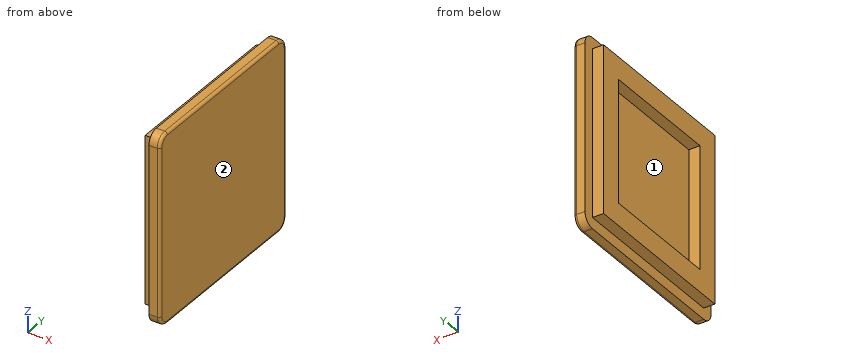
Autodesk Inventor part; units mm, degrees
ref_plane "YZ Plane" through (0, 0, 0) normal (1, 0, 0) x (0, 1, 0)
ref_plane "XZ Plane" through (0, 0, 0) normal (0, 1, 0) x (-1, 0, 0)
ref_plane "XY Plane" through (0, 0, 0) normal (0, 0, 1) x (1, 0, 0)
sketch "Sketch1" plane through (0, 0, 0) normal (1, 0, 0) x (0, 1, 0)
  line L0 (-7.5, 8.5) -> (7.5, 8.5)
  line L1 (8.5, 7.5) -> (8.5, -7.5)
  line L2 (7.5, -8.5) -> (-7.5, -8.5)
  line L3 (-8.5, -7.5) -> (-8.5, 7.5)
  line L4 (-8.5, 8.5) -> (8.5, -8.5) construction
  line L5 (8.5, 8.5) -> (-8.5, -8.5) construction
  line L6 (-7.5, 7.5) -> (7.5, 7.5)
  line L7 (7.5, 7.5) -> (7.5, -7.5)
  line L8 (7.5, -7.5) -> (-7.5, -7.5)
  line L9 (-7.5, -7.5) -> (-7.5, 7.5)
  line L10 (-7.5, 7.5) -> (7.5, -7.5) construction
  line L11 (7.5, 7.5) -> (-7.5, -7.5) construction
  line L12 (-5.5, 5.5) -> (5.5, 5.5)
  line L13 (5.5, 5.5) -> (5.5, -5.5)
  line L14 (5.5, -5.5) -> (-5.5, -5.5)
  line L15 (-5.5, -5.5) -> (-5.5, 5.5)
  line L16 (-5.5, 5.5) -> (5.5, -5.5) construction
  line L17 (5.5, 5.5) -> (-5.5, -5.5) construction
  arc A0 (8.5, 7.5) -> (7.5, 8.5) centre (7.5, 7.5) ccw
  arc A1 (-7.5, 8.5) -> (-8.5, 7.5) centre (-7.5, 7.5) ccw
  arc A2 (-8.5, -7.5) -> (-7.5, -8.5) centre (-7.5, -7.5) ccw
  arc A3 (7.5, -8.5) -> (8.5, -7.5) centre (7.5, -7.5) ccw
  point P0 (0, 0)
  dimension "d0" = 17
  dimension "d1" = 17
  dimension "d2" = 15
  dimension "d3" = 15
  dimension "d4" = 11
  dimension "d5" = 11
  dimension "d12" = 1
extrude "Extrusion3" add sketch "Sketch1" along normal blind 1 contours L0 A0 L1 A3 L2 A2 L3 A1 | L6 L7 L8 L9 | L12 L13 L14 L15
extrude "Extrusion4" add sketch "Sketch1" against normal blind 1 contours L6 L7 L8 L9
fillet "Fillet3" radius 0.25 8 edges at (1, 8.2071, 8.2071) (1, 0, 8.5) (1, -8.2071, 8.2071) (1, -8.5, 0) (1, -8.2071, -8.2071) (1, 0, -8.5) (1, 8.2071, -8.2071) (1, 8.5, 0)
properties part number "cube-inlay-red"
Geometry: final body of the model. Coordinates: model frame, mm. Face numbers are marked on the shaded views. Coordinates: 2 decimals unless noted, no trailing zeros. Order: outer loops, then holes, each group sorted by start corner. A loop starts at its lowest first (then second) coordinate and runs counter-clockwise, first axis right, second up.
1) Ray query, probe 1 along Y at (x, z) = (-0.75, 4.5); probe 2 along X at (y, z) = (-2.75, 3.5). Return the intervals inside material, ascending.
Result sheet:
probe 1: y = -7.5 to -5.5, 5.5 to 7.5
probe 2: x = 0 to 1
2) Section A-A (x = -0.3). Return loops of the section in (y, z), then the cut area to 3 significant figures.
Result sheet:
outline: (-7.5, -7.5) - (7.5, -7.5) - (7.5, 7.5) - (-7.5, 7.5) - close; hole (-5.5, -5.5) - (5.5, -5.5) - (5.5, 5.5) - (-5.5, 5.5) - close
area: 104 mm2
3) Draft query along Y for the marked faces 1 and 2. Return one class per face: released by +Y, released by -Y, zero draft, split by the parting line, or undercut.
Result sheet:
face 1: undercut
face 2: zero draft
4) First-contact query: P1, Ø3.5, axis at y = -1, z = 2.5, coming from the -X side; P2, Ø0.5, axis at x = -0.5, y = 2, coming from the -Z side; P3, Ø0.5, axis at x = -0.5, z = 1, coming from the +Y side. Flat tips, straight axial feed; report the tip coordinate or a pass-through.
Result sheet:
P1: stops at x = 0
P2: stops at z = -7.5
P3: stops at y = 7.5
5) Section C-C (y = -6.5). Return loops of the section in (x, z).
Result sheet:
outline: (-1, -7.5) - (0, -7.5) - (0, -8.5) - (0.75, -8.5) arc R0.25 ccw to (1, -8.25) - (1, 8.25) arc R0.25 ccw to (0.75, 8.5) - (0, 8.5) - (0, 7.5) - (-1, 7.5) - close
6) Section B-B (z = 5). Return loops of the section in (x, y), then the cut area to 3 significant figures.
Result sheet:
outline: (-1, -7.5) - (0, -7.5) - (0, -8.5) - (0.75, -8.5) arc R0.25 ccw to (1, -8.25) - (1, 8.25) arc R0.25 ccw to (0.75, 8.5) - (0, 8.5) - (0, 7.5) - (-1, 7.5) - (-1, 5.5) - (0, 5.5) - (0, -5.5) - (-1, -5.5) - close
area: 21.0 mm2
